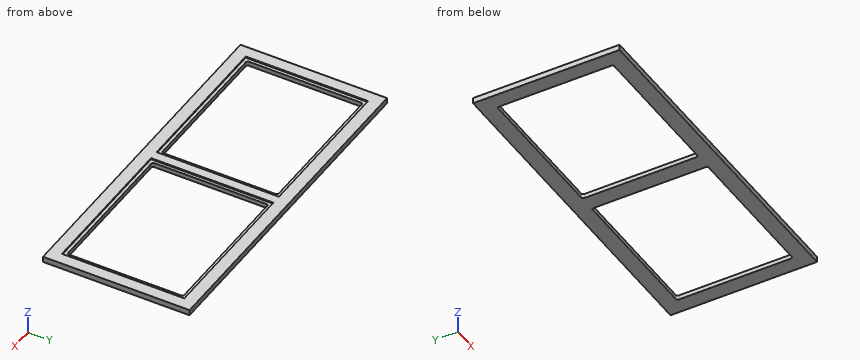
from build123d import *

# Parameters (mm, degrees)
SKETCH_W        = 1064
SKETCH_H        = 460
PAD_DEPTH       = 18
POCKET003_DEPTH = 18.001
SKETCH005_W     = 480
SKETCH005_H     = 384
POCKET_DEPTH    = 4


with BuildPart() as part:
    # Sketch → Pad (new body)
    with BuildSketch(Plane.XY):
        with Locations((-532, 230)):
            Rectangle(SKETCH_W, SKETCH_H)
    extrude(amount=PAD_DEPTH)

    # Sketch004 → Pocket003 (cut, through all)
    with BuildSketch(Plane(origin=(0, 0, 0), x_dir=(1, 0, 0), z_dir=(0, 0, -1))):
        with BuildLine():
            Line((-54.35, -412), (-500.65, -412))
            ThreePointArc((-507, -405.65), (-505.140128, -410.140128), (-500.65, -412))
            Line((-507, -54.35), (-507, -405.65))
            ThreePointArc((-500.65, -48), (-505.140128, -49.859872), (-507, -54.35))
            Line((-54.35, -48), (-500.65, -48))
            ThreePointArc((-48, -54.35), (-49.859872, -49.859872), (-54.35, -48))
            Line((-48, -405.65), (-48, -54.35))
            ThreePointArc((-54.35, -412), (-49.859872, -410.140128), (-48, -405.65))
        make_face()
        with BuildLine():
            Line((-557, -54.35), (-557, -405.65))
            ThreePointArc((-563.35, -412), (-558.859872, -410.140128), (-557, -405.65))
            Line((-563.35, -412), (-1009.65, -412))
            ThreePointArc((-1016, -405.65), (-1014.140128, -410.140128), (-1009.65, -412))
            Line((-1016, -405.65), (-1016, -54.35))
            ThreePointArc((-1009.65, -48), (-1014.140128, -49.859872), (-1016, -54.35))
            Line((-1009.65, -48), (-563.35, -48))
            ThreePointArc((-557, -54.35), (-558.859872, -49.859872), (-563.35, -48))
        make_face()
    extrude(amount=-POCKET003_DEPTH, mode=Mode.SUBTRACT)

    # Sketch005 (on Face5 of Pocket003) → Pocket (cut)
    with BuildSketch(Plane.XY.offset(18)):
        with Locations((-277, 230)):
            Rectangle(SKETCH005_W, SKETCH005_H)
        with Locations((-787, 230)):
            Rectangle(SKETCH005_W, SKETCH005_H)
    extrude(amount=-POCKET_DEPTH, mode=Mode.SUBTRACT)


solid = part.part
Geometry: final body of the model. Coordinates: model frame, mm. Round coordinates to 2 decimals unless told otherwise and drop trailing zeros. Write each loop counter-clockwise with the first axis right and the second up, starting at its lowest first coordinate (ties: lowest second). Pieces come first, ordered by that corner, then holes. Notation, with made-up numbers: M -39,40 L -21,40 A11 ccw -21,57 Z; hole C 71.25,47 d3. An arc over 180 degrees is marked long. Write item = value, one per line.
Item 1: Section query C-C on z = 11.25. Return loops of the section in (x, y), then the cut area to 3 significant figures.
Findings:
outline = M -1064,0 L 0,0 L 0,460 L -1064,460 Z; hole M -1016,54.35 A6.35 ccw -1009.65,48 L -563.35,48 A6.35 ccw -557,54.35 L -557,405.65 A6.35 ccw -563.35,412 L -1009.65,412 A6.35 ccw -1016,405.65 Z; hole M -507,54.35 A6.35 ccw -500.65,48 L -54.35,48 A6.35 ccw -48,54.35 L -48,405.65 A6.35 ccw -54.35,412 L -500.65,412 A6.35 ccw -507,405.65 Z
area = 155,000 mm^2
Item 2: Section query A-A on y = 252. Return loops of the section in (x, z), then the cut area to 3 significant figures.
Findings:
outline = M -1064,0 L -1016,0 L -1016,14 L -1027,14 L -1027,18 L -1064,18 Z; M -557,0 L -507,0 L -507,14 L -517,14 L -517,18 L -547,18 L -547,14 L -557,14 Z; M -48,0 L 0,0 L 0,18 L -37,18 L -37,14 L -48,14 Z
area = 2,460 mm^2
Item 3: Section query B-B on x = -150. Return loops of the section in (y, z), then the cut area to 3 significant figures.
Findings:
outline = M 0,0 L 48,0 L 48,14 L 38,14 L 38,18 L 0,18 Z; M 412,0 L 460,0 L 460,18 L 422,18 L 422,14 L 412,14 Z
area = 1,650 mm^2
Item 4: Material intervals for line 1 along X through (y, z) = (358, 12.25); line 2 along X through (y, z) = (178, 15.25); line 3 along Y through (x, z) = (-629, 1), sorted ascending. Write a range as [from, to].
Findings:
line_1 = [-1064, -1016], [-557, -507], [-48, 0]
line_2 = [-1064, -1027], [-547, -517], [-37, 0]
line_3 = [0, 48], [412, 460]
